```python
from build123d import *

# Parameters (mm, degrees)
F1_DEPTH = 5
F2_W     = 3
F2_H     = 10
F3_DEPTH = 1.5
F4_R     = 0.5
F6_START = -0.75
F5_R     = 3.3
F6_DEPTH = 3.5


# Not quite as in the source:
# - a feature names something its author has since deleted; it is built from what else it names


with BuildPart() as f1:
    # F0 (on Top) → F1 (new body)
    with BuildSketch(Plane.XY):
        with BuildLine():
            Line((-6, -5), (6, -5))
            ThreePointArc((6, -5), (8.8284271247, -3.8284271247), (10, -1))
            Line((10, -1), (10, 1))
            ThreePointArc((10, 1), (8.8284271247, 3.8284271247), (6, 5))
            Line((6, 5), (-6, 5))
            ThreePointArc((-6, 5), (-8.8284271247, 3.8284271247), (-10, 1))
            Line((-10, 1), (-10, -1))
            ThreePointArc((-10, -1), (-8.8284271247, -3.8284271247), (-6, -5))
        make_face()
    extrude(amount=F1_DEPTH)

    # F2 (on face) → F3 (cut)
    with BuildSketch(Plane.XY.offset(5)):
        with Locations((-3.5, 0)):
            Rectangle(F2_W, F2_H)
    extrude(amount=-F3_DEPTH, mode=Mode.SUBTRACT)

    # F4
    f4_edges = [f1.edges().sort_by_distance(p)[0] for p in [
        (-3.5, -5, 3.5),
        (-3.5, 5, 3.5),
        (2, 5, 5),
        (2, -5, 5),
        (-10, 0, 5),
        (-8.828427, 3.828427, 5),
        (-8.828427, -3.828427, 5),
        (-5.5, 5, 5),
        (-5.5, -5, 5),
        (8.828427, -3.828427, 5),
        (10, 0, 5),
        (8.828427, 3.828427, 5),
    ]]
    fillet(f4_edges, radius=F4_R)

    # F5 (on face) → F6 (cut)
    with BuildSketch(Plane(origin=(0, 0, 0), x_dir=(1, 0, 0), z_dir=(0, 0, -1)).offset(F6_START)):
        with Locations((4.7, 0)):
            Circle(F5_R)
    extrude(amount=-F6_DEPTH, mode=Mode.SUBTRACT)


solid = f1.part
```
Can you work these out from the model? Positions are in its coordinate system, mm. A direction names the side the tool comes from. Round coordinates to 2 decimals unless told otherwise and drop trailing zeros. Loops run counter-clockwise (first coordinate to the right, second up) from the corner with the lowest first, then second, coordinate; pieces in that order, holes last. Notation, with made-up numbers: M 62,83 L 110,83 A16 ccw 110,101 Z; hole C 44,84 d9. An arc over 180 degrees is marked long. Write item = value, one per line. Start each with the question number.
(1) Suppose I cut it at B-B on y = 0. Write out the boundary of the cut face in (x, z), plus the area to 3 significant figures.
(2) Which directions (+Z, -Z, +X, -X, +Y, -Y) give clear straight access to the entire face, cutting with the end or side of a thin tool? Please do faces 1 (the face through (10, 0, 2)), 2 (the face through (7.85, -0.99, 2.48)).
(3) Suppose I cut it at C-C on z = 2.8. Write out the boundary of the cut face in (x, y), plus the area to 3 significant figures.
(4) I'm going to push flat-ended pins straight in: P1, Ø2, axis at x = 7.5, z = 2.5, coming from the -Y side; P2, Ø1.6, axis at y = -2.5, z = 4, coming from the -X side. Where does each tip first touch, or does it pass through?
(5) Suppose I cut it at A-A on x = 4.7. Write out the boundary of the cut face in (y, z).
(6) I need wall thicknesses on line 1 along Y through (x, z) = (4.7, 3.05); line 2 along X through (y, z) = (0, 1.95); line 3 along Z through (x, y) = (4.25, -1.5). Which ranges of each line are inside material? Lowest first, please.
(7) If we mould it in two halves opening along X, with no side actions, what happens to faces 3 (the face through (0, 0, 0)), 4 (the face through (-4, 0, 3.5)), 5 (the face through (-10, 0, 2))? For each: released by +X, released by -X, zero draft, split by the parting line, or undercut.
Answer block:
q1.outline = M -10,0 L 10,0 L 10,4.5 A0.5 ccw 9.5,5 L -2,5 L -2,3.5 L -5,3.5 L -5,5 L -9.5,5 A0.5 ccw -10,4.5 Z; hole M 1.4,0.75 L 8,0.75 L 8,4.25 L 1.4,4.25 Z
q1.area = 72.3 mm²
q2.face_1 = +Z, -Z, +X, +Y, -Y
q2.face_2 = none
q3.outline = M -10,-1 A4 ccw -6,-5 L 6,-5 A4 ccw 10,-1 L 10,1 A4 ccw 6,5 L -6,5 A4 ccw -10,1 Z; hole C 4.7,0 d6.6
q3.area = 152 mm²
q4.P1 = -4.97
q4.P2 = -9.94
q5.outline = M -5,0 L 5,0 L 5,4.5 A0.5 ccw 4.5,5 L -4.5,5 A0.5 ccw -5,4.5 Z; hole M -3.3,0.75 L 3.3,0.75 L 3.3,4.25 L -3.3,4.25 Z
q6.line_1 = -5 to -3.3, 3.3 to 5
q6.line_2 = -10 to 1.4, 8 to 10
q6.line_3 = 0 to 0.75, 4.25 to 5
q7.face_3 = zero draft
q7.face_4 = undercut
q7.face_5 = released by -X
